Could you check a few things on this drawing? It's one solid part, dimensions in mm from its lowest x, y, z. A direction names the side the tool comes from. Coordinates: 2 decimals unless noted, no trailing zeros. Loops run counter-clockwise (first coordinate to the right, second up) from the corner with the lowest first, then second, coordinate; pieces in that order, holes last. Notation, with made-up numbers: M 80.25,-16.5 L 130.25,-16.5 A8 cw 130.25,-11.5 Z; hole C 69,-29 d6. An arc over 180 degrees is marked long. Use one line per item in the form item = value. Start each with the question number.
(1) Will these pins go through, and if not, where does the flat tip stop? P1, Ø2, axis at y = 5.5, z = 15.5, coming from the -X side; P2, Ø1, axis at x = 19.5, y = 5.5, coming from the -Z side; P3, Ø1.5, axis at x = 6.5, z = 24, coming from the -Y side; P4, Ø1, axis at x = 20, y = 4, coming from the +Z side.
(2) On a 3-axis mill with a long thin cutter (end or side, diameter ignored), from which of +Z, -Z, +X, -X, +Y, -Y can I reach the whole of each face in a straight line? I mean the marked faces 1 and 2. Say none if no direction works.
(3) Imagine slicing it at C-C, the plane y = 7. Please give me the cut outline in (x, z), and give its area (3 significant figures).
(4) Please list where these lines run through material, in increasing order: L1, parallel to Z at x = 16, y = 0.3; L2, parallel to Z at x = 16, y = 2; L3, parallel to Y at x = 9, z = 10.
(5) Imagine slicing it at D-D, the plane x = 6.5. Please give me the cut outline in (y, z), and give its area (3 significant figures).
(6) Thinking about a two-plate mould opening in X: for the marked faces 3, 4, 5 and 6, which applies, +X half, -X half, draft (parallel to the pull), parting line (faces both ways), or undercut?
(7) Imagine slicing it at B-B, the plane z = 16. Please give me the cut outline in (x, y), and give its area (3 significant figures).
(8) Imagine slicing it at A-A, the plane x = 16. Please give me the cut outline in (y, z), and give its area (3 significant figures).
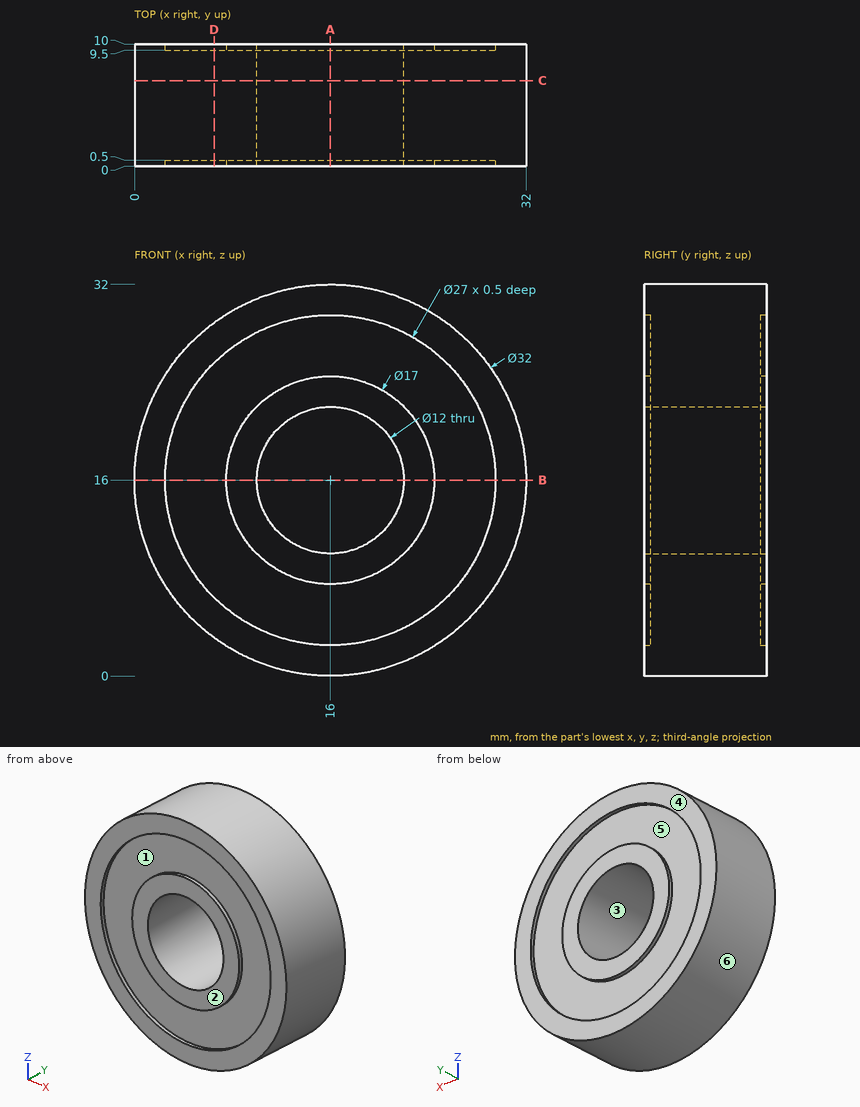
Answer:
q1.P1 = 0
q1.P2 = 0.28
q1.P3 = 0.5
q1.P4 = 31.61
q2.face_1 = -Y
q2.face_2 = +Z, -Z, +X, -X, -Y
q3.outline = C 16,16 d32; hole C 16,16 d12
q3.area = 691 mm²
q4.L1 = 0 to 2.5, 7.5 to 10, 22 to 24.5, 29.5 to 32
q4.L2 = 0 to 10, 22 to 32
q4.L3 = 0.5 to 9.5
q5.outline = M 0,3.13 L 10,3.13 L 10,6.41 L 9.5,6.41 L 9.5,25.59 L 10,25.59 L 10,28.87 L 0,28.87 L 0,25.59 L 0.5,25.59 L 0.5,6.41 L 0,6.41 Z
q5.area = 238 mm²
q6.face_3 = undercut
q6.face_4 = draft
q6.face_5 = undercut
q6.face_6 = parting line
q7.outline = M 0,0 L 2.5,0 L 2.5,0.5 L 7.5,0.5 L 7.5,0 L 10,0 L 10,10 L 7.5,10 L 7.5,9.5 L 2.5,9.5 L 2.5,10 L 0,10 Z; M 22,0 L 24.5,0 L 24.5,0.5 L 29.5,0.5 L 29.5,0 L 32,0 L 32,10 L 29.5,10 L 29.5,9.5 L 24.5,9.5 L 24.5,10 L 22,10 Z
q7.area = 190 mm²
q8.outline = M 0,0 L 10,0 L 10,2.5 L 9.5,2.5 L 9.5,7.5 L 10,7.5 L 10,10 L 0,10 L 0,7.5 L 0.5,7.5 L 0.5,2.5 L 0,2.5 Z; M 0,22 L 10,22 L 10,24.5 L 9.5,24.5 L 9.5,29.5 L 10,29.5 L 10,32 L 0,32 L 0,29.5 L 0.5,29.5 L 0.5,24.5 L 0,24.5 Z
q8.area = 190 mm²
